Here's how the part is built. I have some questions about the finished solid (model axes, mm). A direction names the side the tool comes from. Give positions to 0.01 mm unless a question says otherwise; leave off trailing zeros. Write each loop counter-clockwise with the first axis right and the second up, starting at its lowest first coordinate (ties: lowest second). Pieces come first, ordered by that corner, then holes. Notation, with made-up numbers: (29, 86) -> (74, 86) arc R10 cw to (74, 95) -> close; hole circle Ø3 at (-10.75, 16.25). An arc over 180 degrees is marked (long way). Use CSV: the item, a comma, the result in double quotes. Start each with the question number.
(1) If we mould it in two halves opening along X, with no side actions, what happens to faces 1 (the flat face through (-61, 27, 0)), 2 (the flat face through (-96.057, 50.016, 0.783)), 3 (the flat face through (-114.447, 21.236, 0.783))? For each: pulls with the +X half, pulls with the -X half, needs draft (parallel to the pull), parting line crosses it, or undercut.
(2) Which directions (+Z, -Z, +X, -X, +Y, -Y) give clear straight access to the entire face, cutting with the end or side of a thin tool? Please do faces 4 (the flat face through (-112.375, 15.703, 0.783)), 5 (the cylindrical face through (-156.84, -4.54, 0.78)), 6 (the flat face through (-42.339, 49.745, 0.783)).
(3) Suppose I cut it at A-A on x = -70.5. List the corners of the cut face in (y, z) for me.
(4) I need wall thicknesses on L1, parallel to X at y = 19, z = 1.1; L2, parallel to Y at x = 0, z = 0.95; L3, parallel to X at y = 4, z = 1.4. Which ranges of each line are inside material? Lowest first, please. Write a range as [from, to].
(5) For pin 1 Ø0.8 at (x, z) = (-48.5, 0.5) entering from +Y, with a flat end and sliding along its axis, tell me the tip position at first contact or that it passes through.
(6) Suppose I cut it at B-B on x = -96. List the corners of the cut face in (y, z) for me, plus the area to 3 significant figures.
(7) Suppose I cut it at D-D on z = 0.55. Give the number of separate pieces and of enclosed holes in the cut face, plus the area to 3 significant figures.
(8) Suppose I cut it at C-C on y = 7.5. List the corners of the cut face in (x, z) for me.
Autodesk Inventor part; units mm, degrees
ref_plane "YZ Plane" through (0, 0, 0) normal (1, 0, 0) x (0, 1, 0)
ref_plane "XZ Plane" through (0, 0, 0) normal (0, 1, 0) x (-1, 0, 0)
ref_plane "XY Plane" through (0, 0, 0) normal (0, 0, 1) x (1, 0, 0)
sketch "Sketch1" plane through (0, 0, 0) normal (0, 0, 1) x (1, 0, 0)
  circle A0 centre (0, 0) radius 2.0955
  arc A1 (0, -6.35) -> (2.9931, -5.6004) centre (0, 0) ccw
  arc A2 (-158.75, 0) -> (-152.4, -6.35) centre (-152.4, 0) ccw
  line L0 (-152.4, -6.35) -> (0, -6.35)
  line L1 (-158.75, 28.575) -> (-158.75, 22.225)
  circle A3 centre (-12.7, 2.3813) radius 2.1844
  circle A4 centre (-152.4, 2.3813) radius 2.1844
  circle A5 centre (0, 41.275) radius 2.0955
  circle A6 centre (34.925, 53.975) radius 2.0955
  arc A7 (39.6875, 53.9822) -> (34.6082, 58.727) centre (34.925, 53.975) ccw
  arc A8 (0, -6.35) -> (39.6875, 53.9822) centre (-25.8638, 53.8832) ccw
  circle A9 centre (-12.7, 50.8) radius 2.0955
  arc A10 (-13.0168, 55.552) -> (-16.9032, 53.0393) centre (-12.7, 50.8) ccw
  circle A11 centre (-28.5752, 41.2702) radius 2.0955
  arc A12 (-32.5685, 46.65) -> (-16.9032, 53.0393) centre (-28.5752, 59.2579) ccw
  line L2 (-32.5685, 46.65) -> (-52.3875, 52.9272)
  line L3 (34.6082, 58.727) -> (-13.0168, 55.552)
  line L4 (-52.3875, 52.9272) -> (-140.9672, 47.0219)
  line L5 (-153.0722, 41.582) -> (-123.825, 28.0141)
  line L6 (-123.825, 28.0141) -> (-126.4972, 22.2538)
  line L7 (-80.9625, 34.6421) -> (-80.9625, 29.8796)
  line L8 (20.6375, 29.8796) -> (20.6375, 34.6421)
  line L9 (-116.1342, 17.4463) -> (-112.7125, 25.1339)
  line L10 (-112.7125, 25.1339) -> (-32.3729, 25.1339)
  line L11 (-7.5532, 25.1339) -> (18.2795, 25.1339)
  line L12 (7.9375, 14.0071) -> (1.0071, 14.0071)
  line L13 (-23.8127, 14.0071) -> (-108.7205, 14.0071)
  line L14 (-80.9625, 29.8796) -> (-36.0239, 29.8796)
  line L15 (-20.1488, 29.8796) -> (20.6375, 29.8796)
  line L16 (-23.8127, 14.0071) -> (-32.3729, 25.1339)
  line L17 (-36.0239, 29.8796) -> (-39.6879, 34.6421)
  line L18 (20.6375, 34.6421) -> (-23.8127, 34.6421)
  line L19 (-39.6879, 34.6421) -> (-80.9625, 34.6421)
  line L20 (1.0071, 14.0071) -> (-7.5532, 25.1339)
  line L21 (-20.1488, 29.8796) -> (-23.8127, 34.6421)
  arc A13 (-140.9672, 47.0219) -> (-153.0722, 41.582) centre (-139.7, 28.0141) ccw
  arc A14 (-156.8393, 36.3296) -> (-158.75, 28.0141) centre (-139.7, 28.0141) ccw
  line L22 (-108.7205, 14.0071) -> (-116.1342, 17.4463)
  line L23 (-126.4972, 22.2538) -> (-156.8393, 36.3296)
  line L24 (-158.75, 3.7399) -> (-147.5087, 12.7329)
  line L25 (-158.75, 3.7399) -> (-142.9797, 16.3561)
  line L26 (-142.9797, 16.3561) -> (-158.75, 16.3561)
  line L27 (-158.75, 28.0141) -> (-158.75, 16.3561)
  line L28 (-158.75, 3.7399) -> (-158.75, 0)
  arc A15 (7.9375, 14.0071) -> (18.2795, 25.1339) centre (3.9598, 28.0739) ccw
  dimension "d36" = 4.191
  dimension "d52" = 4.3688
  dimension "d53" = 4.3688
  dimension "d54" = 4.191
  dimension "d57" = 4.191
  dimension "d59" = 4.191
  dimension "d63" = 4.191
  dimension "d66" = 4.7625
  dimension "d70" = 20.1958
extrude "Extrusion1" add sketch "Sketch1" along normal blind 1.5875
equation "\"BendRadius\" = Thickness"
equation "\"BendReliefWidth\" = Thickness"
equation "\"BendReliefDepth\" = 0.5 * Thickness"
equation "\"CornerReliefSize\" = 4 * Thickness"
equation "\"MinimumRemnant\" = 2 * Thickness"
equation "\"TransitionRadius\" = BendRadius"
equation "\"JacobiRadiusSize\" = BendRadius"
equation "\"GapSize\" = Thickness"
properties part number "sled" material "Acetal Resin, White"
Geometry says:
1,face 1,"needs draft"
1,face 2,"pulls with the -X half"
1,face 3,"undercut"
2,face 4,"+Z, -Z"
2,face 5,"+Z, -Z, -X, -Y"
2,face 6,"+Z, -Z, +Y"
3,outline,"(-6.35, 0) -> (14.01, 0) -> (14.01, 1.59) -> (-6.35, 1.59) -> close; (25.13, 0) -> (29.88, 0) -> (29.88, 1.59) -> (25.13, 1.59) -> close; (34.64, 0) -> (51.72, 0) -> (51.72, 1.59) -> (34.64, 1.59) -> close"
4,L1,"[-158.75, -115.44], [-27.65, -2.83], [15.42, 29.64]"
4,L2,"[-6.35, -2.1], [2.1, 15.32], [25.13, 29.88], [34.64, 39.18], [43.37, 56.42]"
4,L3,"[-158.42, -153.87], [-150.93, -14.17], [-11.23, 16.66]"
5,pin 1,"y = 51.82"
6,outline,"(-6.35, 0) -> (14.01, 0) -> (14.01, 1.59) -> (-6.35, 1.59) -> close; (25.13, 0) -> (50.02, 0) -> (50.02, 1.59) -> (25.13, 1.59) -> close"
6,area,"71.8 mm²"
7,separate pieces,"1"
7,enclosed holes,"11"
7,area,"8,760 mm²"
8,outline,"(-154.05, 0) -> (20.46, 0) -> (20.46, 1.59) -> (-154.05, 1.59) -> close"
